Geometry check sheet. Reference: the model listing, model coordinates, mm. A direction names the side the tool comes from. Coordinates: 2 decimals unless noted, no trailing zeros. Loops run counter-clockwise (first coordinate to the right, second up) from the corner with the lowest first, then second, coordinate; pieces in that order, holes last. Notation, with made-up numbers: (78.5, -11.5) - (123.5, -11.5) arc R21 ccw to (123.5, 19.5) - close; hole circle Ø9 at (32.25, 78.25). An arc over 180 degrees is marked (long way). One line per item, written item: value.
from build123d import *

# Parameters (mm, degrees)
F1_DEPTH = 12.7
F2_DEPTH = 1.27
F3_R     = 7.62


# Not quite as in the source:
# - a feature names something its author has since deleted; it is built from what else it names


with BuildPart() as f1:
    # F0 (on Front) → F1 (new body, symmetric)
    with BuildSketch(Plane.XZ):
        Polygon((-46.139964322, 1.8357970985), (-49.8430333048, 1.8357970985), (-49.8430333048, -1.9742029015), (-24.4430333048, -1.9742029015), (-24.4430333048, 1.8357970985), (-33.8560845901, 1.8357970985), align=None)
    extrude(amount=F1_DEPTH, both=True)

    # F0 (on Front) → F2 (join, symmetric)
    with BuildSketch(Plane.XZ):
        Polygon((-31.998090446, 36.4759527147), (-46.139964322, 1.8357970985), (-33.8560845901, 1.8357970985), (-24.9732534132, 36.2684692324), align=None)
    extrude(amount=F2_DEPTH, both=True)

    # F3
    f3_edges = [f1.edges().sort_by_distance(p)[0] for p in [
        (-31.99809, 0, 36.475953),
    ]]
    fillet(f3_edges, radius=F3_R)


solid = f1.part
(1) Go/stop test with flat-tipped pins: pin 1 Ø1.5 at (x, z) = (-37, 23) entering from -Y; pin 2 Ø6.5 at (x, z) = (-32, 18) entering from +Y; pin 3 Ø2 at (x, y) = (-41.5, 4) entering from +Z. Record where each tip stops, or that it passes through.
Reply:
pin 1: y = -1.27
pin 2: y = 1.27
pin 3: z = 1.84
(2) Cross-section at A-A on x = -29. Record the cut outline in (y, z).
Reply:
outline: (-12.7, -1.97) - (12.7, -1.97) - (12.7, 1.84) - (-12.7, 1.84) - close; (-1.27, 20.66) - (1.27, 20.66) - (1.27, 36.04) - (-1.27, 36.04) - close
(3) Material ranges on probe 1 along Z at (x, y) = (-38.75, -3); probe 2 along Y at (x, z) = (-39.25, 3); probe 3 along X at (y, z) = (-0.25, 33), recorded low to high. Write a range as from..to.
Reply:
probe 1: -1.97..1.84
probe 2: -1.27..1.27
probe 3: -33.23..-25.82
(4) Access from +Z, -Z, +X, -X, +Y, -Y to the whole of each face (thin tool, end or side, straight path). Record for faces 1 (the face through (-36, -1.27, 15)), 2 (the face through (-36, 1.27, 15)), 3 (the face through (-37, 12.7, 0)).
Reply:
face 1: +Z, +X, -X, -Y
face 2: +Z, +X, -X, +Y
face 3: +Z, -Z, +X, -X, +Y
(5) Cross-section at B-B on y = 4.25. Record the cut outline in (x, z), and give its area (3 significant figures).
Reply:
outline: (-49.84, -1.97) - (-24.44, -1.97) - (-24.44, 1.84) - (-49.84, 1.84) - close
area: 96.8 mm2
(6) Release check for a two-part mould opening along Z. For faces 4 (the face through (-49.843, 0, 0)), 5 (the face through (-29.477, -0.018, 18.811)), 6 (the face through (-39.98, -0.02, 16.92)) record: pulls with the +Z half, pulls with the -Z half, needs draft (parallel to the pull), parting line crosses it, or undercut.
Reply:
face 4: needs draft
face 5: undercut
face 6: pulls with the +Z half
(7) Cross-section at C-C on x = -34.5. Record the cut outline in (y, z), and give its area (3 significant figures).
Reply:
outline: (-12.7, -1.97) - (12.7, -1.97) - (12.7, 1.84) - (1.27, 1.84) - (1.27, 30.35) - (-1.27, 30.35) - (-1.27, 1.84) - (-12.7, 1.84) - close
area: 169 mm2
(8) Cross-section at D-D on z = 29.5. Record the cut outline in (x, y).
Reply:
outline: (-34.85, -1.27) - (-26.72, -1.27) - (-26.72, 1.27) - (-34.85, 1.27) - close
